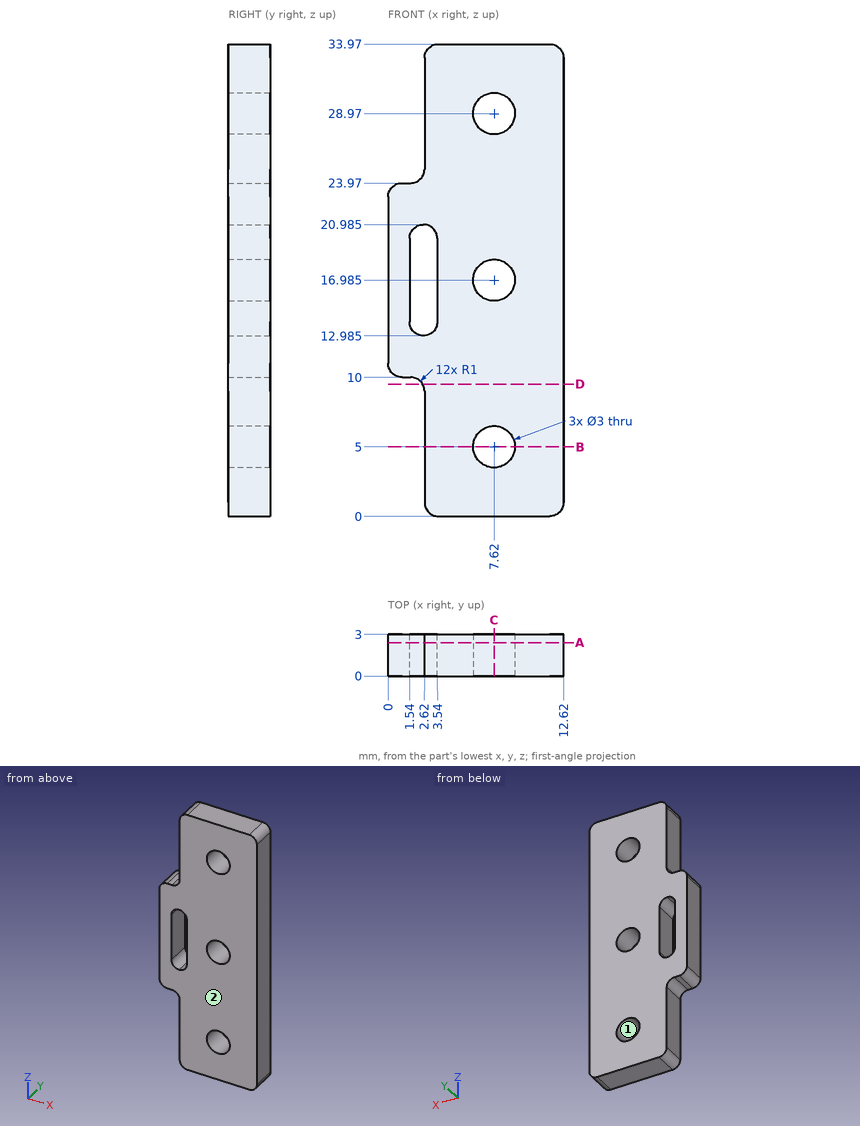
The drawing under review shows one solid part. Ordinate dimensions are in mm from its lowest x, y, z. Round coordinates to 2 decimals unless told otherwise and drop trailing zeros. Loops run counter-clockwise (first coordinate to the right, second up) from the corner with the lowest first, then second, coordinate; pieces in that order, holes last. Notation, with made-up numbers: M 70.25,37.5 L 76.25,37.5 A25 cw 76.25,70.5 Z; hole C 12.25,-37 d2. An arc over 180 degrees is marked long. Answer as CSV lines item,"result". Start each with the question number.
Item 1: Consider section C-C (x = 7.62). Write out the cut boundary in (y, z) (3 decimals), then the cut area to 3 significant figures.
Item 2: Insertion check: P1, Ø0.9, axis at y = 1.5, z = 5.5, coming from the -X side; P2, Ø0.5, axis at x = 1.5, y = 1.5, coming from the +Z side. Each pin has a flat end and moves straight along its axis. Give the tip position at first contact, or say it passes through.
Item 3: Wall thickness on line 1 (Z direction, x = 7.75, y = 2.75); line 2 (X direction, y = 1.1, z = 5); line 3 (Z direction, x = 6.5, y = 0.75): over which ranges is each line inside the solid? List them lowest first. Write a range as [from, to].
Item 4: Consider section D-D (z = 9.5). Write out the cut boundary in (x, y).
Item 5: Consider section A-A (y = 2.4). State how many separate pieces and enclosed holes the cut face has, then the cut area to 3 significant figures.
Item 6: Consider section B-B (z = 5). Write out the cut boundary in (x, y).
Item 7: Mouldability with a two-part tool opening along X and no side actions: class the marked faces 1 and 2 as released by +X, released by -X, zero draft, split by the parting line, or undercut.
Answer:
1,outline,"M 0,0 L 3,0 L 3,3.5 L 0,3.5 Z; M 0,6.5 L 3,6.5 L 3,15.485 L 0,15.485 Z; M 0,18.485 L 3,18.485 L 3,27.47 L 0,27.47 Z; M 0,30.47 L 3,30.47 L 3,33.97 L 0,33.97 Z"
1,area,"74.9 mm^2"
2,P1,"stops at x = 2.62"
2,P2,"stops at z = 23.98"
3,line 1,"z = [0, 3.51], [6.49, 15.49], [18.48, 27.48], [30.46, 33.97]"
3,line 2,"x = [2.62, 6.12], [9.12, 12.62]"
3,line 3,"z = [0, 4], [6, 15.99], [17.98, 27.97], [29.97, 33.97]"
4,outline,"M 2.49,0 L 12.62,0 L 12.62,3 L 2.49,3 Z"
5,separate pieces,"1"
5,enclosed holes,"4"
5,area,"339 mm^2"
6,outline,"M 2.62,0 L 6.12,0 L 6.12,3 L 2.62,3 Z; M 9.12,0 L 12.62,0 L 12.62,3 L 9.12,3 Z"
7,face 1,"undercut"
7,face 2,"zero draft"
